Work out the finished part from the listing and answer in its coordinate system (mm). Face numbers are marked on the shaded views. A direction names the side the tool comes from. Coordinates: 2 decimals unless noted, no trailing zeros. Order: outer loops, then holes, each group sorted by start corner. A loop starts at its lowest first (then second) coordinate and runs counter-clockwise, first axis right, second up. Notation, with made-up numbers: (22.25, -13) -> (53.25, -13) arc R12 ccw to (53.25, 10) -> close; hole circle Ø10 at (-8, -34.75). An arc over 180 degrees is marked (long way). Use one line per item in the form item = value.
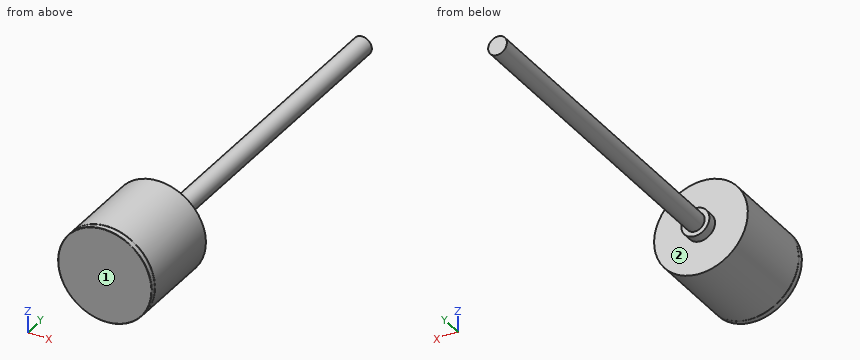
from build123d import *

# Parameters (mm, degrees)
SKETCH_1_R      = 5
EXTRUDE_1_DEPTH = 0.6
FILLET_1_R      = 0.05
FILLET_2_R      = 0.05
SKETCH_2_R      = 5
EXTRUDE_2_DEPTH = 9
SKETCH_3_R      = 1.5
EXTRUDE_3_DEPTH = 1
SKETCH_4_R      = 1
EXTRUDE_4_DEPTH = 35


with BuildPart() as part:
    # Sketch 1 → Extrude 1 (new body)
    with BuildSketch(Plane(origin=(0, 0, 0), x_dir=(1, 0, 0), z_dir=(0, 1, 0))):
        with Locations(Location((0, 0, 0), (0, 0, 270))):
            Circle(SKETCH_1_R)
    extrude(amount=EXTRUDE_1_DEPTH)

    # Fillet 1
    fillet_1_edges = [part.edges().sort_by_distance(p)[0] for p in [
        (0, 0.6, -5),
    ]]
    fillet(fillet_1_edges, radius=FILLET_1_R)

    # Fillet 2
    fillet_2_edges = [part.edges().sort_by_distance(p)[0] for p in [
        (0, 0, -5),
    ]]
    fillet(fillet_2_edges, radius=FILLET_2_R)

    # Sketch 2 → Extrude 2 (add)
    with BuildSketch(Plane(origin=(0, 0.6, 0), x_dir=(1, 0, 0), z_dir=(0, 1, 0))):
        with Locations(Location((0, 0, 0), (0, 0, 270))):
            Circle(SKETCH_2_R)
    extrude(amount=EXTRUDE_2_DEPTH)

    # Sketch 3 → Extrude 3 (add)
    with BuildSketch(Plane(origin=(0, 9.6, 0), x_dir=(1, 0, 0), z_dir=(0, 1, 0))):
        with Locations(Location((0, 0, 0), (0, 0, 270))):
            Circle(SKETCH_3_R)
    extrude(amount=EXTRUDE_3_DEPTH)

    # Sketch 4 → Extrude 4 (add)
    with BuildSketch(Plane(origin=(0, 10.6, 0), x_dir=(1, 0, 0), z_dir=(0, 1, 0))):
        with Locations(Location((0, 0, 0), (0, 0, 270))):
            Circle(SKETCH_4_R)
    extrude(amount=EXTRUDE_4_DEPTH)


solid = part.part
(1) Section C-C on y = 20 is taken. Write down the section's boundary in (x, z).
Data:
outline = circle Ø2 at (0, 0)
(2) Section B-B on x = 0 is taken. Write down the section's boundary in (y, z).
Data:
outline = (0, -4.95) arc R0.05 ccw to (0.05, -5) -> (0.55, -5) arc R0.05 ccw to (0.6, -4.95) -> (0.6, -5) -> (9.6, -5) -> (9.6, -1.5) -> (10.6, -1.5) -> (10.6, -1) -> (45.6, -1) -> (45.6, 1) -> (10.6, 1) -> (10.6, 1.5) -> (9.6, 1.5) -> (9.6, 5) -> (0.6, 5) -> (0.6, 4.95) arc R0.05 ccw to (0.55, 5) -> (0.05, 5) arc R0.05 ccw to (0, 4.95) -> close
(3) Each of these flat-tipped pins is pushed along its axis until it touches: P1, Ø6, axis at y = 10.5, z = 1.5, coming from the +X side; P2, Ø3, axis at x = -2, z = 2, coming from the +Y side; P3, Ø1.5, axis at y = 33, z = 2, coming from the +X side; P4, Ø1, axis at y = 29.5, z = -0.5, coming from the +X side. Where does it stop, or does it pass through?
Data:
P1 = 5
P2 = 10.6
P3 = through
P4 = 1
(4) Straight lines are drawn through the part: line 1 along Y through (x, z) = (-0.75, 2.75); line 2 along X through (y, z) = (3.5, -0.25); line 3 along Z through (x, y) = (0.75, 25). For each, find the intervals that lie inside material, in ascending order.
Data:
line_1 = 0 to 9.6
line_2 = -4.99 to 4.99
line_3 = -0.66 to 0.66
(5) Section D-D on y = 4 is taken. Write down the section's boundary in (x, z).
Data:
outline = circle Ø10 at (0, 0)
(6) Which of the six approach directions +Z, -Z, +X, -X, +Y, -Y give full straight-line access (tool end or side, diameter ignored) to the marked faces 1 and 2?
Data:
face_1 = +Z, -Z, +X, -X, -Y
face_2 = +Y
(7) Section A-A on z = 0 is taken. Write down the section's boundary in (x, y).
Data:
outline = (-5, 0.05) arc R0.05 ccw to (-4.95, 0) -> (4.95, 0) arc R0.05 ccw to (5, 0.05) -> (5, 0.55) arc R0.05 ccw to (4.95, 0.6) -> (5, 0.6) -> (5, 9.6) -> (1.5, 9.6) -> (1.5, 10.6) -> (1, 10.6) -> (1, 45.6) -> (-1, 45.6) -> (-1, 10.6) -> (-1.5, 10.6) -> (-1.5, 9.6) -> (-5, 9.6) -> (-5, 0.6) -> (-4.95, 0.6) arc R0.05 ccw to (-5, 0.55) -> close
